Geometry: see drawing. Coordinates: mm, zero at the bounding-box minimum. Round coordinates to 2 decimals unless told otherwise and drop trailing zeros. Write each loop counter-clockwise with the first axis right and the second up, starting at its lowest first coordinate (ties: lowest second). Pieces come first, ordered by that corner, then holes. Notation, with made-up numbers: (63.25, 64) -> (112.25, 64) arc R25 ccw to (112.25, 82) -> close; hole circle Ø7 at (32.5, 43). An arc over 180 degrees is marked (long way). Use CSV: the item, a comma, the result in double quotes.
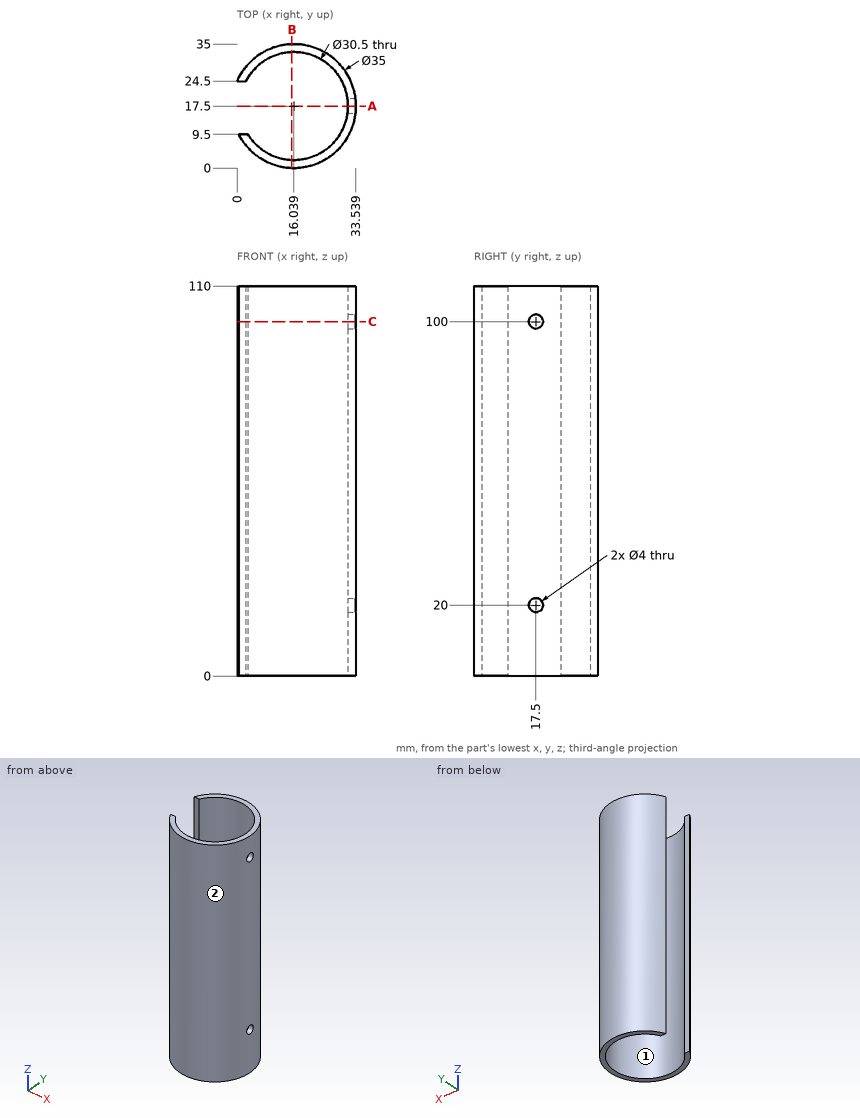
Item 1: First-contact query: pin 1 Ø6.5 at (y, z) = (17.5, 20) entering from +X; pin 2 Ø2 at (x, z) = (1.5, 44) entering from -Y; pin 3 Ø6 at (x, y) = (26.5, 15.5) entering from -Z; pin 4 Ø4 at (x, z) = (10, 37.5) entering from -Y. Flat tips, straight axial feed; report the tip coordinate or a pass-through.
Worked answers:
pin 1,"stops at x = 33.54"
pin 2,"stops at y = 6.41"
pin 3,"passes through"
pin 4,"stops at y = 0.47"
Item 2: Section query A-A on y = 17.5. Return the cut outline in (x, z), plus the area to 4 significant figures.
Worked answers:
outline,"(31.29, 0) -> (33.54, 0) -> (33.54, 18) -> (31.29, 18) -> close; (31.29, 22) -> (33.54, 22) -> (33.54, 98) -> (31.29, 98) -> close; (31.29, 102) -> (33.54, 102) -> (33.54, 110) -> (31.29, 110) -> close"
area,"229.5 mm²"
Item 3: Section query C-C on z = 100. Return the cut outline in (x, y).
Worked answers:
outline,"(0, 24.5) -> (2.49, 24.5) arc R15.25 cw to (31.16, 19.5) -> (33.42, 19.5) arc R17.5 ccw to start; (0.47, 9.5) arc R17.5 ccw to (33.42, 15.5) -> (31.16, 15.5) arc R15.25 cw to (3.06, 9.5) -> close"
Item 4: Section query B-B on x = 15.5. Return the cut outline in (y, z).
Worked answers:
outline,"(0.01, 0) -> (2.26, 0) -> (2.26, 110) -> (0.01, 110) -> close; (32.74, 0) -> (34.99, 0) -> (34.99, 110) -> (32.74, 110) -> close"
Item 5: Line query: line 1 (Z direction, x = 32.2, y = 17.5); line 2 (Z direction, x = 32, y = 17); line 3 (Y direction, x = 19, z = 28.5). Output: solid intervals per line, ascending.
Worked answers:
line 1,"z = 0 to 18, 22 to 98, 102 to 110"
line 2,"z = 0 to 18.06, 21.94 to 98.06, 101.94 to 110"
line 3,"y = 0.25 to 2.54, 32.46 to 34.75"
Item 6: Pull-direction query (X, two-part tool) for the marked faces 1 and 2; classes: +X half, -X half, draft (parallel to the pull), parting line (faces both ways), or undercut.
Worked answers:
face 1,"undercut"
face 2,"parting line"
